from build123d import *

# Parameters (mm, degrees)
BOSS_EXTRUDE1_DEPTH       = 6.35
M5_CLEARANCE_HOLE1_D      = 5.5
M5_CLEARANCE_HOLE1_DEPTH  = 12.7
M5_CLEARANCE_HOLE1_TIP    = 1.652366702
F_6_CLEARANCE_HOLE2_D     = 3.7973
F_6_CLEARANCE_HOLE2_DEPTH = 12.7
F_6_CLEARANCE_HOLE2_TIP   = 1.140824014
M5_CLEARANCE_HOLE2_D      = 5.5
M5_CLEARANCE_HOLE2_DEPTH  = 12.7
M5_CLEARANCE_HOLE2_TIP    = 1.652366702
FILLET1_R                 = 6.35
SKETCH8_R                 = 8
CUT_EXTRUDE1_DEPTH        = 6.35


with BuildPart() as part:
    # Sketch1 → Boss-Extrude1 (new body)
    with BuildSketch(Plane(origin=(0, 0, 0), x_dir=(1, 0, 0), z_dir=(0, 1, 0))):
        Polygon((-228.6, 12.7), (228.6, 12.7), (285.75, 12.7), (285.75, -59.055), (228.6, -59.055), (228.6, -12.7), (-228.6, -12.7), (-228.6, -38.1), (-279.4, -38.1), (-279.4, -12.7), (-292.1, -12.7), (-292.1, 12.7), (-279.4, 12.7), align=None)
    extrude(amount=BOSS_EXTRUDE1_DEPTH)

    # M5 Clearance Hole1
    with Locations(Plane(origin=(0, 6.35, 0), x_dir=(1, 0, 0), z_dir=(0, 1, 0))):
        with Locations((-270.167891819, -6.003039934), (-260.696960066, -28.867891819), (-237.832108181, -19.396960066), (-260.696960066, 3.467891819), (-247.303039934, 3.467891819), (-237.832108181, -6.003039934), (-270.167891819, -19.396960066), (-247.303039934, -28.867891819)):
            Hole(M5_CLEARANCE_HOLE1_D / 2, depth=M5_CLEARANCE_HOLE1_DEPTH)
            with Locations((0, 0, -(M5_CLEARANCE_HOLE1_DEPTH + M5_CLEARANCE_HOLE1_TIP / 2))):  # 118° drill point
                Cone(0, M5_CLEARANCE_HOLE1_D / 2, M5_CLEARANCE_HOLE1_TIP, mode=Mode.SUBTRACT)

    # #6 Clearance Hole2
    with Locations(Plane(origin=(0, 0, -12.7), x_dir=(-1, 0, 0), z_dir=(0, 0, -1))):
        with Locations((279.4, 3.175), (215.9, 3.175), (0, 3.175), (-215.9, 3.175), (-276.225, 3.175)):
            Hole(F_6_CLEARANCE_HOLE2_D / 2, depth=F_6_CLEARANCE_HOLE2_DEPTH)
            with Locations((0, 0, -(F_6_CLEARANCE_HOLE2_DEPTH + F_6_CLEARANCE_HOLE2_TIP / 2))):  # 118° drill point
                Cone(0, F_6_CLEARANCE_HOLE2_D / 2, F_6_CLEARANCE_HOLE2_TIP, mode=Mode.SUBTRACT)

    # M5 Clearance Hole2
    with Locations(Plane(origin=(0, 6.35, 0), x_dir=(1, 0, 0), z_dir=(0, 1, 0))):
        with Locations((218.475, -17.174999994), (218.475, -37.174999994), (244.475, -27.174999994), (256.475, -3.175), (256.475, -51.175), (236.475, -3.175), (236.475, -51.175), (270.475, -17.174999994), (270.475, -37.174999994)):
            Hole(M5_CLEARANCE_HOLE2_D / 2, depth=M5_CLEARANCE_HOLE2_DEPTH)
            with Locations((0, 0, -(M5_CLEARANCE_HOLE2_DEPTH + M5_CLEARANCE_HOLE2_TIP / 2))):  # 118° drill point
                Cone(0, M5_CLEARANCE_HOLE2_D / 2, M5_CLEARANCE_HOLE2_TIP, mode=Mode.SUBTRACT)

    # Fillet1
    fillet1_edges = [part.edges().sort_by_distance(p)[0] for p in [
        (285.75, 3.175, 59.055),
        (228.6, 3.175, 59.055),
        (228.6, 3.175, 12.7),
        (-228.6, 3.175, 12.7),
        (-228.6, 3.175, 38.1),
        (-279.4, 3.175, 38.1),
        (-279.4, 3.175, 12.7),
        (-292.1, 3.175, 12.7),
    ]]
    fillet(fillet1_edges, radius=FILLET1_R - 0.0001)  # a hair under: the kernel refuses the full size

    # Sketch8 → Cut-Extrude1 (cut)
    with BuildSketch(Plane(origin=(0, 6.35, 0), x_dir=(1, 0, 0), z_dir=(0, 1, 0))):
        with Locations(Location((-254, -12.7, 0), (0, 0, 270))):
            Circle(SKETCH8_R)
        with Locations(Location((244.475, -27.174999994, 0), (0, 0, 270))):
            Circle(SKETCH8_R)
    extrude(amount=-CUT_EXTRUDE1_DEPTH, mode=Mode.SUBTRACT)


solid = part.part
Design review of the part built by this model. Coordinates are the model's own, in mm. Coordinates: 2 decimals unless noted, no trailing zeros. Loops run counter-clockwise (first coordinate to the right, second up) from the corner with the lowest first, then second, coordinate; pieces in that order, holes last. Notation, with made-up numbers: M -34,-37.75 L -11,-37.75 A15 cw -11,-10.75 Z; hole C 37.5,-27.75 d6. An arc over 180 degrees is marked long. Use one line per item in the form item = value.
(1) For line 1 along X through (y, z) = (4.25, 51.5); line 2 along X through (y, z) = (0.5, 25.5); line 3 along Z through (x, y) = (-258.5, 2.25), list the stretches that pass through material, from the lowest coordinate up. Write a range as from..to.
Return value:
line_1 = 228.6..233.74, 239.21..253.74, 259.21..285.75
line_2 = -279.4..-228.6, 228.6..236.65, 252.3..285.75
line_3 = -12.7..-5.12, -1.81..6.09, 19.31..27.21, 30.52..38.1
(2) Consider section A-A (x = 96.5). Write out the cut boundary in (y, z), and give its area (3 significant figures).
Return value:
outline = M 0,-12.7 L 6.35,-12.7 L 6.35,12.7 L 0,12.7 Z
area = 161 mm2
(3) Draft analysis for pull direction X (two halves, no side actions). For faces 1 (the face through (65, 0, 7)), 2 (the face through (-246.068, 3.219, 11.659)), state which applies: pulls with the +X half, pulls with the -X half, needs draft (parallel to the pull), parting line crosses it, or undercut.
Return value:
face_1 = needs draft
face_2 = undercut
(4) Clearance check with flat-ended pins moving along their axes: P1, Ø3, axis at y = 4, z = 37, coming from the -X side; P2, Ø3, axis at x = 276.225, y = 3.175, coming from the -Z side; P3, Ø2, axis at y = 2, z = 40.5, coming from the -X side. State where each tip first meets the part, or that it passes through.
Return value:
P1 = -278.17
P2 = 0.24
P3 = 228.6
